Design review of the part built by this model. Coordinates are the model's own, in mm. Face numbers are marked on the shaded views. A direction names the side the tool comes from. Coordinates: 2 decimals unless noted, no trailing zeros. Write each loop counter-clockwise with the first axis right and the second up, starting at its lowest first coordinate (ties: lowest second). Pieces come first, ordered by that corner, then holes. Notation, with made-up numbers: (51, 7) -> (63, 7) arc R29 cw to (63, 36) -> close; hole circle Ø3 at (12.5, -29). An arc over 180 degrees is marked (long way). Answer in a Markdown table with one row per item. Add a question column.
Item 1: For the marked faces 1, 2, 3 and 4, list the 3-axis set-ups (+Z, -Z, +X, -X, +Y, -Y) from which the entire face can be reached by the end or side of a thin tool; tool diameter is ignored.
Item 2: Take a section at D-D, the plane x = -23.5. Write out the cut boundary in (y, z), and give its area (3 significant figures).
Item 3: Take a section at B-B, the plane y = 59.8. Write out the cut boundary in (x, z), and give its area (3 significant figures).
Item 4: Take a section at C-C, the plane z = -8.75. Write out the cut boundary in (x, y) (3 decimals).
Item 5: Draft analysis for pull direction X (two halves, no side actions). For the marked faces 5, 6 and 7, state which applies: released by +X, released by -X, zero draft, split by the parting line, or undercut.
Item 6: Clearance check with flat-ended pins moving along their axes: P1, Ø8, axis at y = 53, z = 10, coming from the +X side; P2, Ø1.2, axis at y = 1.5, z = -11, coming from the -X side; P3, Ø1.8, axis at x = -3.375, y = 4, coming from the -Z side; P4, Ø21, axis at y = 36, z = 4, coming from the +X side. State where each tip first meets the part, or that it passes through.
Item 7: Take a section at A-A, the plane z = 0. Write out the cut boundary in (x, y) (3 decimals), and give its area (3 significant figures).
Item 8: To check wall thickness, follow line 1 (Z direction, x = -2, y = 59); line 2 (X direction, y = 3, z = -6) (3 decimals); line 3 (Y direction, x = 48, z = -6.5). State the ranges of each line that lie inside material, in increasing order.
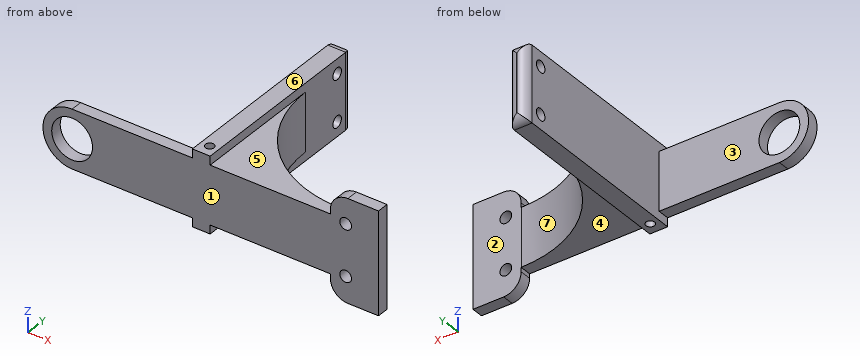
Autodesk Inventor part; units mm, degrees
ref_plane "YZ Plane" through (0, 0, 0) normal (1, 0, 0) x (0, 1, 0)
ref_plane "XZ Plane" through (0, 0, 0) normal (0, 1, 0) x (-1, 0, 0)
ref_plane "XY Plane" through (0, 0, 0) normal (0, 0, 1) x (1, 0, 0)
sketch "Main Sketch" plane through (0, 0, 0) normal (0, 1, 0) x (-1, 0, 0)
  line L0 (-57.375, -12.0472) -> (-57.375, 12.0472)
  line L1 (-57.375, 12.0472) -> (47.625, -10) construction
  line L2 (47.625, 10) -> (-57.375, -12.0472) construction
  circle A0 centre (47.625, 0) radius 7
  arc A1 (47.625, -10) -> (47.625, 10) centre (47.625, 0) ccw
  line L3 (-40.875, 17.5) -> (-57.375, 17.5)
  line L4 (-57.375, 17.5) -> (-57.375, -17.5)
  line L5 (-57.375, -17.5) -> (-40.875, -17.5)
  line L6 (-40.875, 17.5) -> (-57.375, -17.5) construction
  line L7 (-57.375, 17.5) -> (-40.875, -17.5) construction
  line L8 (47.625, -10) -> (-40.875, -10)
  line L9 (-40.875, -17.5) -> (-40.875, -10)
  line L10 (-40.875, 10) -> (-40.875, 17.5)
  line L11 (-40.875, 10) -> (47.625, 10)
  point P0 (0, 0)
  point P1 (-49.125, 0)
  dimension "d3" = 14
  dimension "d4" = 105
  dimension "d13" = 16.5
  dimension "d14" = 35
  dimension "d15" = 0
  dimension "d18" = 20
extrude "Main Extrusion" add sketch "Main Sketch" along normal blind 4
sketch "Screw Holes Sketch" plane through (0, 4, 0) normal (0, 1, 0) x (1, 0, 0)
  circle A0 centre (46.125, -8.75) radius 2
  line L0 (57.375, 17.5) -> (40.875, 17.5)
  line L1 (40.875, -17.5) -> (57.375, -17.5)
  line L2 (35.2664, 0) -> (65.7891, 0)
  line L3 (51.375, -27.0398) -> (51.375, 30.2346) construction
  line L4 (57.375, -17.5) -> (57.375, 17.5)
  line L5 (40.875, -10) -> (40.875, -17.5)
  circle A1 centre (46.125, 8.75) radius 2
  line L6 (51.375, 27.0398) -> (51.375, -30.2346) construction
  point P0 (0, 0)
  dimension "d21" = 4
  dimension "d22" = 35
  dimension "d23" = 6
  dimension "d24" = 5.25
  dimension "d25" = 5.25
  dimension "d26" = 10.5
  dimension "d27" = 8.75
  dimension "d28" = 17.5
extrude "Screw Holes Cut" cut sketch "Screw Holes Sketch" against normal through all
fillet "Smoooooooooooooooooth" radius 6 2 edges at (40.875, 2, -17.5) (40.875, 2, 17.5)
sketch "Side Axel Hole Sketch" plane through (-47.625, 0, 10) normal (0, 0, 1) x (1, 0, 0)
  line L0 (88.5, 4) -> (88.5, 0)
  line L1 (0, 0) -> (0, 4)
  line L2 (44.25, -12.0383) -> (44.25, 22.7681) construction
  line L3 (88.5, 0) -> (0, 0)
  line L4 (0, 4) -> (88.5, 4)
  circle A0 centre (44.25, 4) radius 1.5
  point P0 (47.625, 0)
  dimension "d32" = 88.5
  dimension "d33" = 44.25
  dimension "d34" = 44.25
  dimension "d35" = 4
  dimension "d41" = 3
sketch "Sketch7" plane through (0, 4, 0) normal (0, 1, 0) x (1, 0, 0)
  line L0 (-47.625, -10) -> (40.875, -10) construction
  line L1 (-3.375, -10) -> (-3.375, 33.3565) construction
  line L2 (-0.3194, -13) -> (-6.4306, -13)
  line L3 (-6.4306, -13) -> (-6.4306, 13)
  line L4 (-6.4306, 13) -> (-0.3194, 13)
  line L5 (-0.3194, 13) -> (-0.3194, -13)
  line L6 (-0.3194, -13) -> (-6.4306, 13) construction
  line L7 (-6.4306, -13) -> (-0.3194, 13) construction
  point P0 (0, 0)
  point P1 (-3.375, 0)
  dimension "d47" = 26
extrude "Servo Mount Extrusion" add sketch "Sketch7" along normal blind 62.8 and the other way blind 4
extrude "Side Axel Cut" cut sketch "Side Axel Hole Sketch" along normal through all both and the other way through all contours A0 L4 | L4 A0
sketch "Sketch8" plane through (-6.4306, 4, -10) normal (-1, 0, 0) x (0, 0, 1)
  line L0 (23, 62.8) -> (23, -4) construction
  line L1 (-3, 62.8) -> (23, 62.8) construction
  line L2 (-3, 62.8) -> (-3, -4) construction
  circle A0 centre (2, 55.8) radius 2
  circle A1 centre (18, 55.8) radius 2
  point P0 (10, -4)
  dimension "d54" = 4
  dimension "d55" = 4
  dimension "d56" = 16
  dimension "d57" = 7
  dimension "d58" = 7
  dimension "d59" = 5
  dimension "d60" = 5
extrude "Mount Holes Cut" cut sketch "Sketch8" against normal through all
fillet "Support" radius 41 1 edges at (-0.3194, 4, 0)
fillet "lil hat" radius 3 4 edges at (-0.3194, 66.8, 0) (-3.375, 66.8, -13) (-6.4306, 66.8, 0) (-3.375, 66.8, 13)
properties part number "TapeMeasureBracketSideServo"
Answers:
| question | item | result |
|---|---|---|
| 1 | face 1 | +Z, -Z, +X, -X, -Y |
| 1 | face 2 | +Z, -Z, +X, +Y |
| 1 | face 3 | +Z, -Z, -X, +Y |
| 1 | face 4 | -Z, +Y, -Y |
| 2 | outline | (0, -10) -> (4, -10) -> (4, 10) -> (0, 10) -> close |
| 2 | area | 80.0 mm^2 |
| 3 | outline | (-6.43, -13) -> (-0.32, -13) -> (-0.32, -10) -> (-6.43, -10) -> close; (-6.43, -6) -> (-0.32, -6) -> (-0.32, 6) -> (-6.43, 6) -> close; (-6.43, 10) -> (-0.32, 10) -> (-0.32, 13) -> (-6.43, 13) -> close |
| 3 | area | 110 mm^2 |
| 4 | outline | (-52.466, 0) -> (44.125, 0) -> (44.125, 4) -> (40.681, 4) arc R41 cw to (-0.319, 45) -> (-0.319, 57.946) -> (-6.431, 57.946) -> (-6.431, 4) -> (-52.466, 4) -> close; (-6.431, 61.654) -> (-0.319, 61.654) -> (-0.319, 63.8) arc R3 ccw to (-3.319, 66.8) -> (-3.431, 66.8) arc R3 ccw to (-6.431, 63.8) -> close; (48.125, 0) -> (57.375, 0) -> (57.375, 4) -> (48.125, 4) -> close; hole circle Ø3 at (-3.375, 4) |
| 5 | face 5 | undercut |
| 5 | face 6 | zero draft |
| 5 | face 7 | released by +X |
| 6 | P1 | stops at x = -0.32 |
| 6 | P2 | stops at x = -6.43 |
| 6 | P3 | passes through |
| 6 | P4 | stops at x = 4.61 |
| 7 | outline | (-57.625, 0) -> (-54.625, 0) -> (-54.625, 4) -> (-57.625, 4) -> close; (-40.625, 0) -> (57.375, 0) -> (57.375, 4) -> (40.681, 4) arc R41 cw to (-0.319, 45) -> (-0.319, 63.8) arc R3 ccw to (-3.319, 66.8) -> (-3.431, 66.8) arc R3 ccw to (-6.431, 63.8) -> (-6.431, 4) -> (-40.625, 4) -> close; hole circle Ø3 at (-3.375, 4) |
| 7 | area | 1,140 mm^2 |
| 8 | line 1 | z = -13 to -9.83, -6.17 to 6.17, 9.83 to 13 |
| 8 | line 2 | x = -55.625 to -51.231, -44.019 to -4.493, -2.257 to 57.375 |
| 8 | line 3 | y = 0 to 4 |
